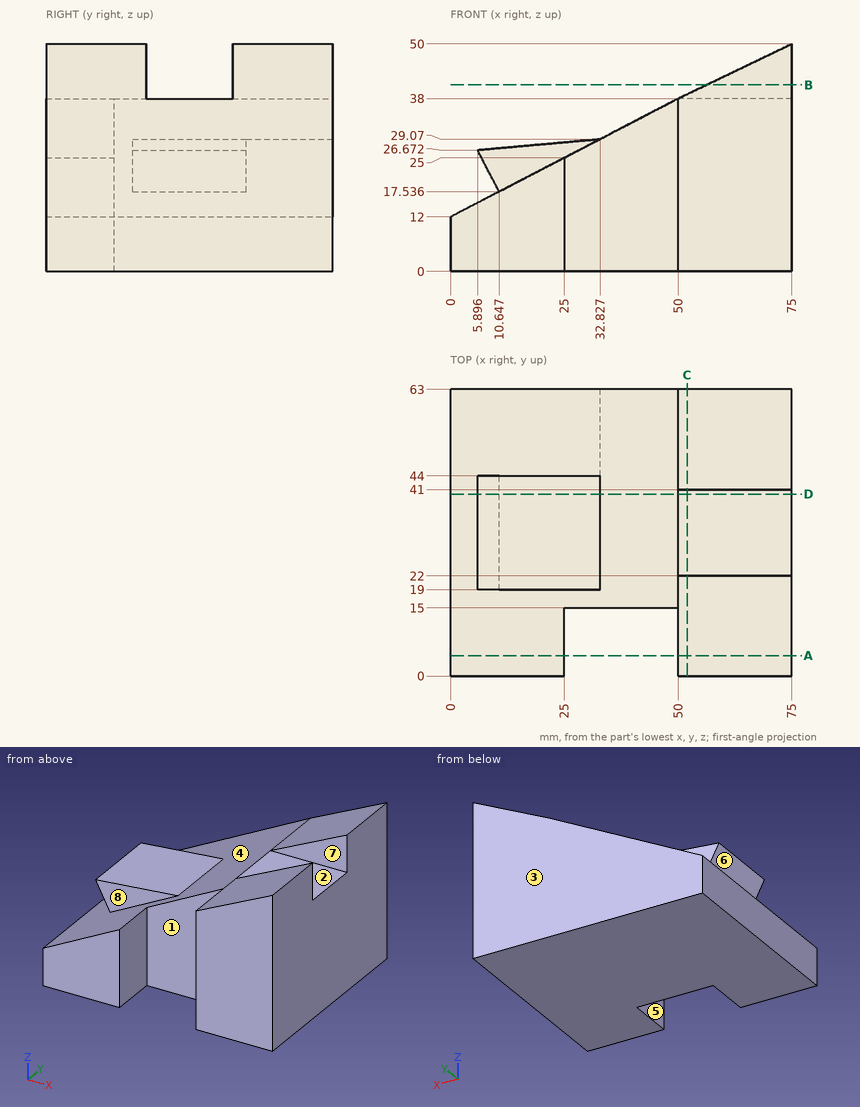
Check sheet for the drawn part. Datum: minimum x, y, z corner. Units: mm. A direction names the side the tool comes from. Round coordinates to 2 decimals unless told otherwise and drop trailing zeros. Write each loop counter-clockwise with the first axis right and the second up, starting at its lowest first coordinate (ties: lowest second). Pieces come first, ordered by that corner, then holes. Notation, with made-up numbers: (79.5, -30.5) -> (83.5, -30.5) arc R21 ccw to (83.5, -0.5) -> close; hole circle Ø9 at (-37, 88.25). An arc over 180 degrees is marked (long way). One line per item, written item: value. Start each with the question number.
(1) Draft check along Y on the marked faces 1, 2, 3 and 4. Enter one of: +Y half, -Y half, draft (parallel to the pull), parting line (faces both ways), or undercut.
(2) Cross-section at D-D, the plane y = 40. Record the cut outline in (x, z).
(3) Access from +Z, -Z, +X, -X, +Y, -Y to the whole of each face (thin tool, end or side, straight path). Record for the marked faces 5, 6, 7 and 8.
(4) Cross-section at B-B, the plane z = 41. Record the cut outline in (x, y).
(5) Cross-section at C-C, the plane x = 52. Record the cut outline in (y, z).
(6) Go/stop test with flat-tipped pins: pin 1 Ø7.5 at (x, z) = (35, 13) entering from -Y; pin 2 Ø3 at (y, z) = (44.5, 32.5) entering from -X. Record where each tip stops, or that it passes through.
(7) Cross-section at A-A, the plane y = 4.5. Record the cut outline in (x, z).
(8) Scan lines: line 1 (X direction, y = 13, z = 11.5); line 2 (Z direction, x = 61, y = 31.5); line 3 (Y direction, x = 34.5, z = 16). Record each from-to range of solid material in increasing order. Write a range as [from, to].
Answer:
1. face 1: -Y half
1. face 2: undercut
1. face 3: +Y half
1. face 4: draft
2. outline: (0, 0) -> (75, 0) -> (75, 38) -> (50, 38) -> (32.83, 29.07) -> (5.9, 26.67) -> (10.65, 17.54) -> (0, 12) -> close
3. face 5: +Z, -Z, -Y
3. face 6: -X, +Y, -Y
3. face 7: +Z, +X, -X
3. face 8: +Z, -X, -Y
4. outline: (56.25, 0) -> (75, 0) -> (75, 22) -> (56.25, 22) -> close; (56.25, 41) -> (75, 41) -> (75, 63) -> (56.25, 63) -> close
5. outline: (0, 0) -> (63, 0) -> (63, 38.96) -> (41, 38.96) -> (41, 38) -> (22, 38) -> (22, 38.96) -> (0, 38.96) -> close
6. pin 1: y = 15
6. pin 2: x = 36.54
7. outline: (0, 0) -> (25, 0) -> (25, 25) -> (0, 12) -> close; (50, 0) -> (75, 0) -> (75, 50) -> (50, 38) -> close
8. line 1: [0, 25], [50, 75]
8. line 2: [0, 38]
8. line 3: [15, 63]
